```python
from build123d import *

# Parameters (mm, degrees)
SKETCH4_R           = 0.8
BOSS_EXTRUDE2_DEPTH = 38.3
SKETCH6_R           = 0.9
BOSS_EXTRUDE3_DEPTH = 0.2
SKETCH7_R           = 0.75
CUT_EXTRUDE1_DEPTH  = 38.25
SKETCH8_W           = 0.215319984
SKETCH8_H           = 0.113992932
BOSS_EXTRUDE4_DEPTH = 5


with BuildPart() as part:
    # Sketch4 → Boss-Extrude2 (new body)
    with BuildSketch(Plane.XY):
        Circle(SKETCH4_R)
    extrude(amount=BOSS_EXTRUDE2_DEPTH)

    # Sketch6 → Boss-Extrude3 (add)
    with BuildSketch(Plane(origin=(0, 0, 11.45), x_dir=(-1, 0, 0), z_dir=(0, 0, -1))):
        Circle(SKETCH6_R)
    extrude(amount=BOSS_EXTRUDE3_DEPTH)

    # Sketch7 → Cut-Extrude1 (cut)
    with BuildSketch(Plane(origin=(0, 0, 0), x_dir=(-1, 0, 0), z_dir=(0, 0, -1))):
        Circle(SKETCH7_R)
    extrude(amount=-CUT_EXTRUDE1_DEPTH, mode=Mode.SUBTRACT)

    # Sketch8 → Boss-Extrude4 (add)
    with BuildSketch(Plane.XY.offset(38.3)):
        Rectangle(SKETCH8_W, SKETCH8_H)
    extrude(amount=BOSS_EXTRUDE4_DEPTH)


solid = part.part
```
For this review, take the finished solid that the model builds, in its own axes (mm). Coordinates: 2 decimals unless noted, no trailing zeros. Write each loop counter-clockwise with the first axis right and the second up, starting at its lowest first coordinate (ties: lowest second). Pieces come first, ordered by that corner, then holes. Notation, with made-up numbers: (15.5, -26) - (69.5, -26) arc R24 ccw to (69.5, 3) - close; hole circle Ø10 at (12, -25.75). An arc over 180 degrees is marked (long way). Answer in a Markdown table with one row per item. Add a question column.
Q1. For probe 1 along Z at (x, y) = (0.55, -0.65); probe 2 along X at (y, z) = (0, 41), list the stretches that pass through material, from the lowest coordinate up.
Q2. We need section A-A, the plane z = 23.5. State the section outline as (x, y) points, and give its area (3 significant figures).
Q3. For P1, Ø0.9, axis at x = 0, y = 0, coming from the -Z side; P2, Ø0.5, axis at x = 0.5, y = 0, coming from the +Z side, all flat-tipped, find the tip position at first contact; note any pin that passes through.
Answer list:
| question | item | result |
|---|---|---|
| 1 | probe 1 | z = 11.25 to 11.45 |
| 1 | probe 2 | x = -0.11 to 0.11 |
| 2 | outline | circle Ø1.6 at (0, 0); hole circle Ø1.5 at (0, 0) |
| 2 | area | 0.243 mm2 |
| 3 | P1 | stops at z = 38.25 |
| 3 | P2 | stops at z = 38.3 |
